```python
from build123d import *

# Parameters (mm, degrees)
F0_R     = 12.7
F1_DEPTH = 304.8
F3_DEPTH = 25.4
F7_DEPTH = 8.89
F9_DEPTH = 10.795


with BuildPart() as f1:
    # F0 (on Front) → F1 (new body)
    with BuildSketch(Plane.XZ):
        Circle(F0_R)
    extrude(amount=-F1_DEPTH)

    # F2 (on face) → F3 (cut)
    with BuildSketch(Plane.XZ):
        with BuildLine():
            ThreePointArc((3.175, 12.296722), (0, 12.7), (-3.175, 12.296722))
            Line((-3.175, 12.296722), (-3.175, 3.81))
            Line((-3.175, 3.81), (3.175, 3.81))
            Line((3.175, 3.81), (3.175, 12.296722))
        make_face()
        with BuildLine():
            Line((-4.7625, -1.905), (-4.7625, -11.773215))
            ThreePointArc((-4.7625, -11.773215), (0, -12.7), (4.7625, -11.773215))
            Line((4.7625, -11.773215), (4.7625, -1.905))
            Line((4.7625, -1.905), (-4.7625, -1.905))
        make_face()
    extrude(amount=-F3_DEPTH, mode=Mode.SUBTRACT)

    # F6 (on offset) → F7 (cut, through all)
    with BuildSketch(Plane.XY.offset(12.7)):
        with BuildLine():
            Line((-3.175, 25.4), (3.175, 25.4))
            ThreePointArc((3.175, 25.4), (0, 28.575), (-3.175, 25.4))
        make_face()
    extrude(amount=-F7_DEPTH, mode=Mode.SUBTRACT)

    # F8 (on offset) → F9 (cut, through all)
    with BuildSketch(Plane.XY.offset(-12.7)):
        with BuildLine():
            ThreePointArc((4.7625, 25.4), (0, 30.1625), (-4.7625, 25.4))
            Line((-4.7625, 25.4), (4.7625, 25.4))
        make_face()
    extrude(amount=F9_DEPTH, mode=Mode.SUBTRACT)


solid = f1.part
```
CAD build for the part. Positions are in the model's coordinates, mm. A direction names the side the tool comes from. Round coordinates to 2 decimals unless told otherwise and drop trailing zeros. Loops run counter-clockwise (first coordinate to the right, second up) from the corner with the lowest first, then second, coordinate; pieces in that order, holes last. Notation, with made-up numbers: (-16.75, 23.5) - (-9.75, 23.5) arc R9 ccw to (-9.75, 28.5) - close; hole circle Ø3 at (89, -6). An arc over 180 degrees is marked (long way). Return JSON: item names as keys, results as strings. Group by question number.
Q1. Band-saw the part on A-A on x = 0. Give the cut face in (y, z) (1 decimal).
Q2. Tool access for faces 4 (the face through (3.175, 13, 8)), 5 (the face through (0.1, 30.16, -7.38)), 6 (the face through (0, 0, 0)): list every direction of +Z, -Z, +X, -X, +Y, -Y with a clear straight run to the whole face (end or side of a thin tool).
Q3. Band-saw the part on B-B on z = 8. Give the cut face in (x, y) (3 decimals).
Q4. Two-plate mould, pull along X, no slides. Class faces 1 (the face through (0, 304.8, 0)), 2 (the face through (12.114, 150.266, 3.815)), 3 (the face through (-3.175, 13, 8)): +X half, -X half, draft (parallel to the pull), parting line (faces both ways), or undercut.
Q5. Drill centre lines: line 1 along Z through (x, y) = (-1.75, 28) (3 decimals); line 2 along Y through (x, z) = (0.5, -10.75); line 3 along Z through (x, y) = (5.25, 23). Where is each one in solid material? Low to high. Write a range as [from, to].
Q6. Flat gauge pins, fed straight in: pin 1 Ø8 at (y, z) = (9.5, -5.5) entering from +X; pin 2 Ø7 at (x, y) = (-0.5, 13.5) entering from +Z; pin 3 Ø5 at (x, y) = (-7, 228) entering from +Z. Where does each tip first touch, or does it go through?
Q7. Band-saw the part on C-C on y = 231. Give the cut face in (x, z), plus the area to 3 significant figures.
Solutions:
{
 "1": {"outline": "(0, -1.9) - (30.2, -1.9) - (30.2, -12.7) - (304.8, -12.7) - (304.8, 12.7) - (28.6, 12.7) - (28.6, 3.8) - (0, 3.8) - close"},
 "2": {"face 4": "+Z, -Y", "face 5": "-Z, -Y", "face 6": "+Z, -Z, +X, -X, -Y"},
 "3": {"outline": "(-9.864, 0) - (-3.175, 0) - (-3.175, 25.4) arc R3.175 cw to (3.175, 25.4) - (3.175, 0) - (9.864, 0) - (9.864, 304.8) - (-9.864, 304.8) - close"},
 "4": {"face 1": "draft", "face 2": "parting line", "face 3": "undercut"},
 "5": {"line 1": "z = [-1.905, 3.81]", "line 2": "y = [30.14, 304.8]", "line 3": "z = [-11.56, 11.56]"},
 "6": {"pin 1": "stops at x = 12.61", "pin 2": "stops at z = 12.3", "pin 3": "stops at z = 11.88"},
 "7": {"outline": "circle Ø25.4 at (0, 0)", "area": "507 mm^2"}
}
